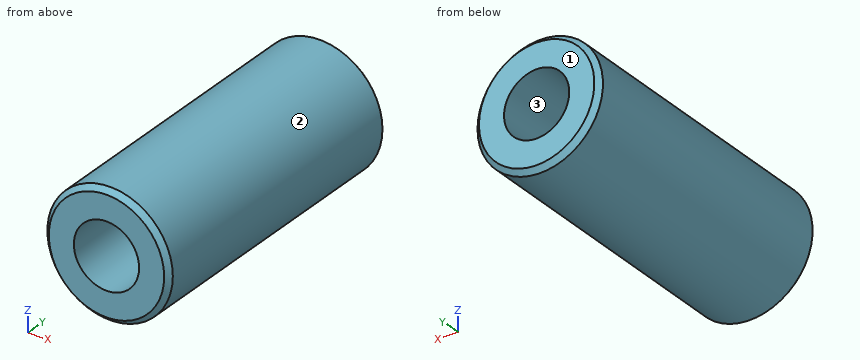
Autodesk Inventor part; units mm, degrees
ref_plane "YZ Plane" through (0, 0, 0) normal (1, 0, 0) x (0, 1, 0)
ref_plane "XZ Plane" through (0, 0, 0) normal (0, 1, 0) x (-1, 0, 0)
ref_plane "XY Plane" through (0, 0, 0) normal (0, 0, 1) x (1, 0, 0)
sketch "スケッチ1" plane through (0, 0, 0) normal (0, 1, 0) x (1, 0, 0)
  circle A0 centre (0, 0) radius 2.5
  circle A1 centre (0, 0) radius 1.3
  dimension "d0" = 5
  dimension "d1" = 2.6
extrude "押し出し1" add sketch "スケッチ1" along normal mid plane 12
chamfer "面取り1" distance 0.2 angle 45 2 edges at (-2.5, 6, 0) (-2.5, -6, 0)
properties part number "ARL-2612E"
The listing builds one solid part. Answer for the finished solid, in the listing's coordinates (mm). Face numbers are marked on the shaded views. Round coordinates to 2 decimals unless told otherwise and drop trailing zeros. Write each loop counter-clockwise with the first axis right and the second up, starting at its lowest first coordinate (ties: lowest second). Pieces come first, ordered by that corner, then holes. Notation, with made-up numbers: (44.5, 75) -> (101.5, 75) arc R18 cw to (101.5, 97) -> close; hole circle Ø7 at (-16, 24). An arc over 180 degrees is marked (long way). Write item = value, one per line.
1) Section B-B on z = 0 is taken. Write down the section's boundary in (x, y), plus the area to 3 significant figures.
Check values:
outline = (-2.5, -5.8) -> (-2.3, -6) -> (-1.3, -6) -> (-1.3, 6) -> (-2.3, 6) -> (-2.5, 5.8) -> close; (1.3, -6) -> (2.3, -6) -> (2.5, -5.8) -> (2.5, 5.8) -> (2.3, 6) -> (1.3, 6) -> close
area = 28.7 mm²
2) Section C-C on y = 2 is taken. Write down the section's boundary in (x, z), plus the area to 3 significant figures.
Check values:
outline = circle Ø5 at (0, 0); hole circle Ø2.6 at (0, 0)
area = 14.3 mm²
3) For a pull along Z with two mould halves and no side action, classify the marked faces 1, 2 and 3 as released by +Z, released by -Z, zero draft, split by the parting line, or undercut.
Check values:
face_1 = zero draft
face_2 = split by the parting line
face_3 = undercut
4) Given pin 1 (1.5 mm diameter, centred on x = -1.5, y = -2.5, fed in from -Z), flat-ended and moving along its own axis, determine where the tip first touches the part or whether it passes through.
Check values:
pin_1 = -2.38
5) Section A-A on x = 0 is taken. Write down the section's boundary in (y, z).
Check values:
outline = (-6, -2.3) -> (-5.8, -2.5) -> (5.8, -2.5) -> (6, -2.3) -> (6, -1.3) -> (-6, -1.3) -> close; (-6, 1.3) -> (6, 1.3) -> (6, 2.3) -> (5.8, 2.5) -> (-5.8, 2.5) -> (-6, 2.3) -> close
6) Straight lines are drawn through the part: line 1 along Z through (x, y) = (0, 1.5); line 2 along Z through (x, y) = (-1, -3.5). For each, find the intervals that lie inside material, in ascending order. Write a range as [from, to].
Check values:
line_1 = [-2.5, -1.3], [1.3, 2.5]
line_2 = [-2.29, -0.83], [0.83, 2.29]
